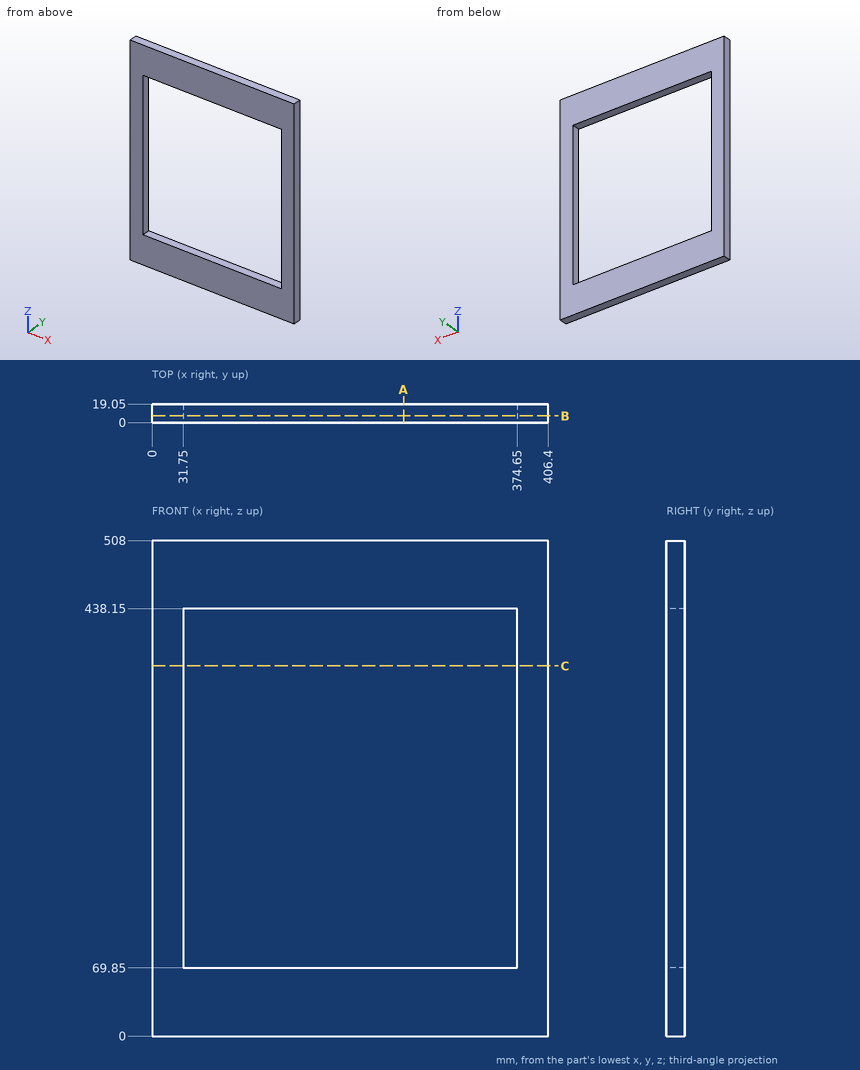
Check sheet for the drawn part. Datum: minimum x, y, z corner. Units: mm. Round coordinates to 2 decimals unless told otherwise and drop trailing zeros. Order: outer loops, then holes, each group sorted by start corner. A loop starts at its lowest first (then second) coordinate and runs counter-clockwise, first axis right, second up.
1. Section check B-B on y = 6.75. Record the cut outline in (x, z).
Final values:
outline: (0, 0) - (406.4, 0) - (406.4, 508) - (0, 508) - close; hole (31.75, 69.85) - (374.65, 69.85) - (374.65, 438.15) - (31.75, 438.15) - close
2. Section check C-C on z = 379.5. Record the cut outline in (x, y).
Final values:
outline: (0, 0) - (31.75, 0) - (31.75, 19.05) - (0, 19.05) - close; (374.65, 0) - (406.4, 0) - (406.4, 19.05) - (374.65, 19.05) - close
3. Thickness scan on L1, parallel to Z at x = 267.5, y = 4.5; L2, parallel to X at y = 7.5, z = 190.5. Record the ranges inside material, lowest first.
Final values:
L1: z = 0 to 69.85, 438.15 to 508
L2: x = 0 to 31.75, 374.65 to 406.4
4. Section check A-A on x = 258. Record the cut outline in (y, z).
Final values:
outline: (0, 0) - (19.05, 0) - (19.05, 69.85) - (0, 69.85) - close; (0, 438.15) - (19.05, 438.15) - (19.05, 508) - (0, 508) - close
